```python
from build123d import *

# Parameters (mm, degrees)
F0_W      = 177.8
F0_H      = 47.6504
F1_DEPTH  = 76.2
F2_R      = 4.7752
F2_R_2    = 1.9812
F3_DEPTH  = 44.45
F5_DEPTH  = 16.002
F7_DEPTH  = 33.528
F9_DEPTH  = 31.7246
F11_DEPTH = 31.7246


# Not quite as in the source:
# - a feature names something its author has since deleted; it is built from what else it names


with BuildPart() as f1:
    # F0 (on Top) → F1 (new body)
    with BuildSketch(Plane.XY):
        with Locations((84.1375, 19.0627)):
            Rectangle(F0_W, F0_H)
    extrude(amount=-F1_DEPTH)

    # F2 (on face) → F3 (cut)
    with BuildSketch(Plane.XZ.offset(4.7625)):
        with Locations((141.5288, -18.1356)):
            Circle(F2_R)
        with Locations((112.9538, -23.8506)):
            Circle(F2_R_2)
        with Locations((91.5416, -15.875)):
            Circle(F2_R_2)
    extrude(amount=-F3_DEPTH, mode=Mode.SUBTRACT)

    # F4 (on face) → F5 (cut)
    with BuildSketch(Plane.XY):
        with BuildLine():
            Line((172.1358, 18.2664336953), (172.1358, 19.8998040895))
            ThreePointArc((172.1358, 19.8998040895), (170.6147547927, 23.7117700549), (166.887268424, 25.4294744577))
            Line((166.887268424, 25.4294744577), (147.1168, 25.4294744577))
            ThreePointArc((147.1168, 25.4294744577), (141.7286463274, 23.1976281303), (139.4968, 17.8094744577))
            Line((139.4968, 17.8094744577), (139.4968, 17.5517135975))
            ThreePointArc((139.4968, 17.5517135975), (140.8917039546, 14.1841175521), (144.2593, 12.7892135975))
            Line((144.2593, 12.7892135975), (165.7858, 12.7892135975))
            ThreePointArc((165.7858, 12.7892135975), (170.2152246474, 14.0735098945), (172.1358, 18.2664336953))
        make_face()
    extrude(amount=-F5_DEPTH, mode=Mode.SUBTRACT)

    # F6 (on face) → F7 (cut)
    with BuildSketch(Plane.XY):
        with BuildLine():
            Line((113.0554, 23.03145), (103.7082, 23.03145))
            ThreePointArc((103.7082, 23.03145), (100.9063600902, 21.8708899098), (99.7458, 19.06905))
            ThreePointArc((99.7458, 19.06905), (100.9063600902, 16.2672100902), (103.7082, 15.10665))
            Line((103.7082, 15.10665), (113.0554, 15.10665))
            ThreePointArc((113.0554, 15.10665), (115.8572399098, 16.2672100902), (117.0178, 19.06905))
            ThreePointArc((117.0178, 19.06905), (115.8572399098, 21.8708899098), (113.0554, 23.03145))
        make_face()
    extrude(amount=-F7_DEPTH, mode=Mode.SUBTRACT)

    # F8 (on face) → F9 (cut)
    with BuildSketch(Plane.XY):
        with BuildLine():
            Line((129.9972, 27.8257), (88.4682, 27.8257))
            ThreePointArc((88.4682, 27.8257), (84.5528083312, 26.2038916688), (82.931, 22.2885))
            Line((82.931, 22.2885), (82.931, 15.8369))
            ThreePointArc((82.931, 15.8369), (84.5528083312, 11.9215083312), (88.4682, 10.2997))
            Line((88.4682, 10.2997), (129.9972, 10.2997))
            ThreePointArc((129.9972, 10.2997), (133.9125916688, 11.9215083312), (135.5344, 15.8369))
            Line((135.5344, 15.8369), (135.5344, 22.2885))
            ThreePointArc((135.5344, 22.2885), (133.9125916688, 26.2038916688), (129.9972, 27.8257))
        make_face()
    extrude(amount=-F9_DEPTH, mode=Mode.SUBTRACT)

    # F10 (on face) → F11 (cut)
    with BuildSketch(Plane.XY):
        with BuildLine():
            Line((142.4686, 23.8379), (134.5240552125, 23.8379))
            ThreePointArc((134.5240552125, 23.8379), (132.2789911822, 22.9079640303), (131.3490552125, 20.6629))
            Line((131.3490552125, 20.6629), (131.3490552125, 15.8877))
            ThreePointArc((131.3490552125, 15.8877), (132.2789911822, 13.6426359697), (134.5240552125, 12.7127))
            Line((134.5240552125, 12.7127), (142.4686, 12.7127))
            ThreePointArc((142.4686, 12.7127), (146.3839916688, 14.3345083312), (148.0058, 18.2499))
            Line((148.0058, 18.2499), (148.0058, 18.3007))
            ThreePointArc((148.0058, 18.3007), (146.3839916688, 22.2160916688), (142.4686, 23.8379))
        make_face()
    extrude(amount=-F11_DEPTH, mode=Mode.SUBTRACT)


solid = f1.part
```
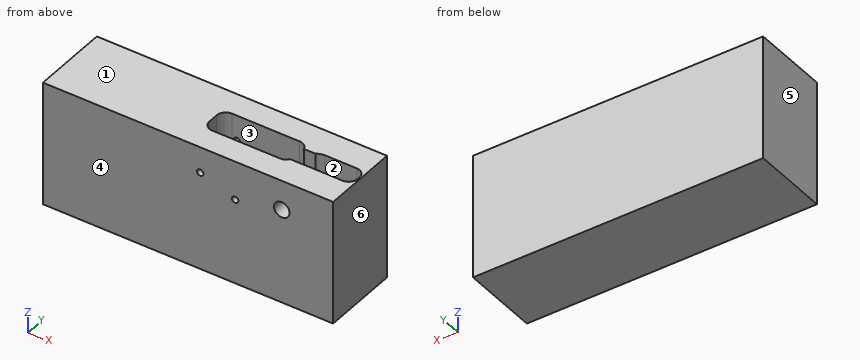
Read the model definition and answer for the solid it produces. Units are mm, in the model's axes. Face numbers are marked on the shaded views. A direction names the side the tool comes from. Give positions to 0.01 mm unless a question says otherwise; leave off trailing zeros. Order: outer loops, then holes, each group sorted by start corner. A loop starts at its lowest first (then second) coordinate and runs counter-clockwise, first axis right, second up.
(1) Given pin 1 (9 mm diameter, centred on x = 112, y = 23, fed in from +Z); pin 2 (4.5 mm diameter, centred on x = 91, z = -16, fed in from -Y); pin 3 (4 mm diameter, centred on x = 107, y = 20, fed in from +Z), each flat-ended and moving along its own axis, determine where each tip first touches the part or whether it passes through.
(2) Straight lines are drawn through the part: L1, parallel to X at y = 7.5, z = -18; L2, parallel to Y at x = 147, z = -12.5; L3, parallel to X at y = 10, z = -16. For each, find the intervals that lie inside material, in ascending order.
(3) Find section A-A (x = 139). Give the vertices of the cut face in (y, z).
(4) Find section C-C (x = 86). Give the vertices of the cut face in (y, z), plus the area to 3 significant figures.
(5) For the marked faces 1 and 2, determine the directions among +Z, -Z, +X, -X, +Y, -Y from which every point of the face is accessible in a straight line to the end or side of a thin tool.
(6) Find section B-B (x = 119). Give the vertices of the cut face in (y, z), plus the area to 3 significant figures.
(7) For a pull along X with two mould halves and no side action, classify the marked faces 3, 4, 5 and 6 as released by +X, released by -X, zero draft, split by the parting line, or undercut.
Result sheet:
1. pin 1: stops at z = -31.72
1. pin 2: stops at y = -4.76
1. pin 3: stops at z = -33.53
2. L1: x = -4.76 to 136.76, 146.3 to 173.04
2. L2: y = -4.76 to 12.79, 25.43 to 42.89
2. L3: x = -4.76 to 89.56, 93.52 to 137.26, 145.8 to 173.04
3. outline: (-4.76, -76.2) - (42.89, -76.2) - (42.89, 0) - (23.84, 0) - (23.84, -14.08) - (39.69, -14.08) - (39.69, -22.19) - (23.84, -22.19) - (23.84, -31.72) - (12.71, -31.72) - (12.71, -22.19) - (-4.76, -22.19) - close; (-4.76, -14.08) - (12.71, -14.08) - (12.71, 0) - (-4.76, 0) - close
4. outline: (-4.76, -76.2) - (42.89, -76.2) - (42.89, 0) - (27.25, 0) - (27.25, -31.72) - (10.88, -31.72) - (10.88, 0) - (-4.76, 0) - close
4. area: 3,110 mm2
5. face 1: +Z, +X, -X, +Y, -Y
5. face 2: +Z
6. outline: (-4.76, -76.2) - (42.89, -76.2) - (42.89, 0) - (27.83, 0) - (27.83, -31.72) - (10.3, -31.72) - (10.3, 0) - (-4.76, 0) - close
6. area: 3,070 mm2
7. face 3: undercut
7. face 4: zero draft
7. face 5: released by -X
7. face 6: released by +X
